For this review, take the finished solid that the model builds, in its own axes (mm). Give positions to 0.01 mm unless a question says otherwise; leave off trailing zeros. Order: outer loops, then holes, each group sorted by start corner. A loop starts at its lowest first (then second) coordinate and runs counter-clockwise, first axis right, second up. Notation, with made-up numbers: (57, 54) - (115, 54) arc R18 ccw to (115, 59) - close; hole circle Ø2 at (-3.75, -20.5). An arc over 180 degrees is marked (long way). Put each result on its own line as item: value. Start each with the question number.
```python
from build123d import *

# Parameters (mm, degrees)
BOSS_EXTRUDE1_DEPTH      = 16.315787
BOSS_EXTRUDE1_DEPTH_BACK = 13.184213
FILLET1_R                = 0.2


with BuildPart() as part:
    # Sketch1 → Boss-Extrude1 (new, two sides: drawn at the far end of the back side and taken through both)
    with BuildSketch(Plane.XY.offset(-BOSS_EXTRUDE1_DEPTH_BACK)):
        Polygon((220, 2.6), (220, 0), (222, 0), (222, 0.6), align=None)
    extrude(amount=BOSS_EXTRUDE1_DEPTH + BOSS_EXTRUDE1_DEPTH_BACK)

    # Fillet1
    fillet1_edges = [part.edges().sort_by_distance(p)[0] for p in [
        (222, 0.3, 16.315787),
        (221, 1.6, 16.315787),
        (220, 1.3, 16.315787),
        (221, 0, 16.315787),
        (222, 0.3, -13.184213),
        (222, 0.6, 1.565787),
        (221, 1.6, -13.184213),
        (220, 2.6, 1.565787),
        (220, 1.3, -13.184213),
        (220, 0, 1.565787),
        (221, 0, -13.184213),
        (222, 0, 1.565787),
    ]]
    fillet(fillet1_edges, radius=FILLET1_R)


solid = part.part
```
1. Add section A-A, the plane z = 13.5. Give the boundary of the cut face in (x, y), then the cut area to 3 significant figures.
2. Wall thickness on line 1 (Y direction, x = 220.25, z = -5.5); line 2 (X direction, y = 0.75, z = 6.5); line 3 (X direction, y = 1.45, z = -10.5): over which ranges is each line inside the solid? List them lowest first. Write a range as from..to.
3. Clearance check with a flat-ended pin moving along its axis: pin 1 (1 mm diameter, centred on x = 221, y = 2, fed in from +Z). State where the tip first meets the part, or that it passes through.
Found:
1. outline: (220, 0.2) arc R0.2 ccw to (220.2, 0) - (221.8, 0) arc R0.2 ccw to (222, 0.2) - (222, 0.52) arc R0.2 ccw to (221.94, 0.66) - (220.34, 2.26) arc R0.2 ccw to (220, 2.12) - close
1. area: 3.13 mm^2
2. line 1: y = 0..2.31
2. line 2: x = 220..221.85
2. line 3: x = 220..221.15
3. pin 1: stops at z = 16.32
